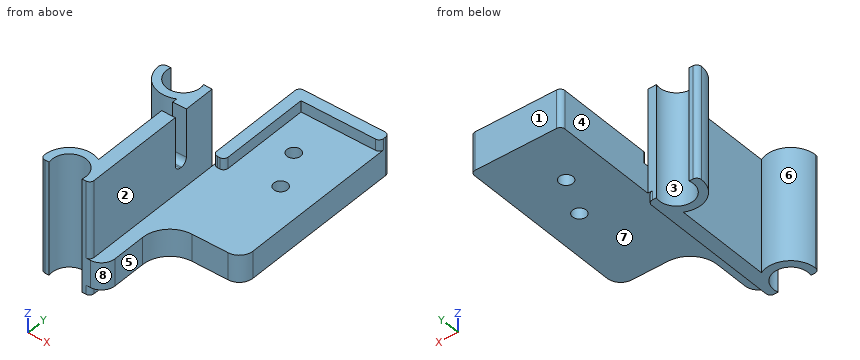
from build123d import *

# Parameters (mm, degrees)
SKETCH1_R           = 3.75
BOSS_EXTRUDE1_DEPTH = 25
FILLET1_R           = 2
SKETCH3_W           = 20
SKETCH3_H           = 19
CUT_EXTRUDE2_DEPTH  = 6
FILLET2_R           = 3
SKETCH7_W           = 32.058329052
SKETCH7_H           = 42.536839165
CUT_EXTRUDE5_DEPTH  = 25
SKETCH10_W          = 12.254265393
SKETCH10_H          = 5.748315633
SKETCH10_W_2        = 13.681746689
SKETCH10_H_2        = 5.503604554
CUT_EXTRUDE6_DEPTH  = 25
SKETCH11_W          = 6
SKETCH11_H          = 56.5
BOSS_EXTRUDE2_DEPTH = 20
CUT_EXTRUDE9_DEPTH  = 3
CUT_EXTRUDE11_DEPTH = 10
BOSS_EXTRUDE3_DEPTH = 2.5
FILLET5_R           = 3
FILLET6_R           = 1
SKETCH17_R          = 1.5
CUT_EXTRUDE12_DEPTH = 10


with BuildPart() as part:
    # Sketch1 → Boss-Extrude1 (new body)
    with BuildSketch(Plane.XY):
        with BuildLine():
            Line((-21, 16.5), (-21, -16.5))
            Line((-21, -16.5), (-16.5, -21))
            Line((-16.5, -21), (16.5, -21))
            Line((16.5, -21), (21, -16.5))
            Line((21, -16.5), (21, 16.5))
            Line((21, 16.5), (16.5, 21))
            Line((16.5, 21), (11.125, 21))
            Line((11.125, 21), (11.125, 18))
            Line((11.125, 18), (10.601020514, 18))
            ThreePointArc((10.601020514, 18), (11.610912703, 11.610912703), (18, 10.601020514))
            Line((18, 10.601020514), (18, -10.601020514))
            ThreePointArc((18, -10.601020514), (11.610912703, -11.610912703), (10.601020514, -18))
            Line((10.601020514, -18), (-10.601020514, -18))
            ThreePointArc((-10.601020514, -18), (-11.610912703, -11.610912703), (-18, -10.601020514))
            Line((-18, -10.601020514), (-18, 10.601020514))
            ThreePointArc((-18, 10.601020514), (-11.610912703, 11.610912703), (-10.601020514, 18))
            Line((-10.601020514, 18), (-11.125, 18))
            Line((-11.125, 18), (-11.125, 21))
            Line((-11.125, 21), (-16.5, 21))
            Line((-16.5, 21), (-21, 16.5))
        make_face()
        with Locations((-15.5, 15.5)):
            Circle(SKETCH1_R, mode=Mode.SUBTRACT)
        with Locations((15.5, 15.5)):
            Circle(SKETCH1_R, mode=Mode.SUBTRACT)
        with Locations((15.5, -15.5)):
            Circle(SKETCH1_R, mode=Mode.SUBTRACT)
        with Locations((-15.5, -15.5)):
            Circle(SKETCH1_R, mode=Mode.SUBTRACT)
    extrude(amount=BOSS_EXTRUDE1_DEPTH)

    # Fillet1
    fillet1_edges = [part.edges().sort_by_distance(p)[0] for p in [
        (-21, -16.5, 12.5),
        (-21, 16.5, 12.5),
        (-16.5, 21, 12.5),
        (-16.5, -21, 12.5),
    ]]
    fillet(fillet1_edges, radius=FILLET1_R)

    # Sketch3 → Cut-Extrude2 (cut)
    with BuildSketch(Plane(origin=(0, -21, 0), x_dir=(-1, 0, 0), z_dir=(0, -1, 0))):
        with Locations((0, -12.5)):
            Rectangle(SKETCH3_W, SKETCH3_H)
    extrude(amount=-CUT_EXTRUDE2_DEPTH, mode=Mode.SUBTRACT)

    # Fillet2
    fillet2_edges = [part.edges().sort_by_distance(p)[0] for p in [
        (10, -19.5, 22),
        (-10, -19.5, 3),
        (-10, -19.5, 22),
        (10, -19.5, 3),
    ]]
    fillet(fillet2_edges, radius=FILLET2_R)

    # Sketch7 → Cut-Extrude5 (cut)
    with BuildSketch(Plane.XY.offset(25)):
        with Locations((-6.029164526, 0.268419582)):
            Rectangle(SKETCH7_W, SKETCH7_H)
    extrude(amount=-CUT_EXTRUDE5_DEPTH, mode=Mode.SUBTRACT)

    # Sketch10 → Cut-Extrude6 (cut)
    with BuildSketch(Plane.XY.offset(25)):
        with Locations((14.872867304, 19.374157817)):
            Rectangle(SKETCH10_W, SKETCH10_H)
        with Locations((14.159126655, -19.251802277)):
            Rectangle(SKETCH10_W_2, SKETCH10_H_2)
    extrude(amount=-CUT_EXTRUDE6_DEPTH, mode=Mode.SUBTRACT)

    # Sketch11 → Boss-Extrude2 (add)
    with BuildSketch(Plane(origin=(21, 0, 0), x_dir=(0, 0, -1), z_dir=(1, 0, 0))):
        with Locations((-5, 11.75)):
            Rectangle(SKETCH11_W, SKETCH11_H)
    extrude(amount=BOSS_EXTRUDE2_DEPTH)

    # Sketch13 → Cut-Extrude9 (cut)
    with BuildSketch(Plane(origin=(21, 0, 0), x_dir=(0, 0, -1), z_dir=(1, 0, 0))):
        with BuildLine():
            Line((-25, 9.5), (-14.35, 9.5))
            ThreePointArc((-14.35, 9.5), (-13.395405845, 9.104594155), (-13, 8.15))
            Line((-13, 8.15), (-13, 7.85))
            ThreePointArc((-13, 7.85), (-13.395405845, 6.895405845), (-14.35, 6.5))
            Line((-14.35, 6.5), (-25, 6.5))
            Line((-25, 6.5), (-25, 9.5))
        make_face()
    extrude(amount=-CUT_EXTRUDE9_DEPTH, mode=Mode.SUBTRACT)

    # Sketch15 → Cut-Extrude11 (cut)
    with BuildSketch(Plane.XY.offset(8)):
        with BuildLine():
            Line((24, -16.5), (24, -6))
            ThreePointArc((24, -6), (25.757359313, -1.757359313), (30, 0))
            Line((30, 0), (41, 0))
            Line((41, 0), (41, -16.5))
            Line((41, -16.5), (24, -16.5))
        make_face()
    extrude(amount=-CUT_EXTRUDE11_DEPTH, mode=Mode.SUBTRACT)

    # Sketch16 → Boss-Extrude3 (add)
    with BuildSketch(Plane.XY.offset(8)):
        Polygon((21, 40), (41, 40), (41, 37.461788715), (23.538211285, 37.478793923), (23.538211285, 16.726527219), (21, 16.726527219), (21, 37.478793923), align=None)
    extrude(amount=BOSS_EXTRUDE3_DEPTH)

    # Fillet5
    fillet5_edges = [part.edges().sort_by_distance(p)[0] for p in [
        (41, 0, 5),
        (24, -16.5, 5),
    ]]
    fillet(fillet5_edges, radius=FILLET5_R)

    # Fillet6
    fillet6_edges = [part.edges().sort_by_distance(p)[0] for p in [
        (10.091673087, 16.5, 12.5),
        (10.091673087, -16.5, 12.5),
        (21, 16.5, 1),
        (21, -16.5, 1),
        (21, 40, 6.25),
        (41, 40, 6.25),
        (21, 16.726527219, 9.25),
        (23.538211285, 16.726527219, 9.25),
        (41, 37.461788715, 9.25),
        (21, -16.5, 16.5),
    ]]
    fillet(fillet6_edges, radius=FILLET6_R)

    # Sketch17 → Cut-Extrude12 (cut)
    with BuildSketch(Plane.XY.offset(8)):
        with Locations((29.574223118, 28.11574528)):
            Circle(SKETCH17_R)
        with Locations((33.574223119, 19.642947284)):
            Circle(SKETCH17_R)
    extrude(amount=-CUT_EXTRUDE12_DEPTH, mode=Mode.SUBTRACT)


solid = part.part
For this review, take the finished solid that the model builds, in its own axes (mm). Face numbers are marked on the shaded views. A direction names the side the tool comes from. Round coordinates to 2 decimals unless told otherwise and drop trailing zeros. Write each loop counter-clockwise with the first axis right and the second up, starting at its lowest first coordinate (ties: lowest second). Pieces come first, ordered by that corner, then holes. Notation, with made-up numbers: (34.25, -16.75) - (79.25, -16.75) arc R19 ccw to (79.25, -2.75) - close; hole circle Ø6 at (67.25, 51.25). An arc over 180 degrees is marked (long way). Use a Markdown table: item, result.
Q1. Clearance check with flat-ended pins moving along their axes: pin 1 (5 mm diameter, centred on x = 26, y = 7, fed in from -Z); pin 2 (2 mm diameter, centred on x = 17.5, z = 6, fed in from -Y); pin 3 (4.5 mm diameter, centred on x = 15.5, y = -15.5, fed in from +Z); pin 4 (3 mm diameter, centred on y = 20, z = 3.5, fed in from -X). State where each tip first meets the part, or that it passes through.
Derived:
| item | result |
|---|---|
| pin 1 | stops at z = 2 |
| pin 2 | stops at y = -13.25 |
| pin 3 | passes through |
| pin 4 | stops at x = 21 |
Q2. The part is to be moulded in two halves that separate along Y. For the marked faces 6, 7 and 8, say which applies: pulls with the +Y half, pulls with the -Y half, needs draft (parallel to the pull), parting line crosses it, or undercut.
Derived:
| item | result |
|---|---|
| face 6 | undercut |
| face 7 | needs draft |
| face 8 | pulls with the -Y half |
Q3. Machinability: for the marked faces 1, 2, 3, 4 and 5, which of the approach directions +Z, -Z, +X, -X, +Y, -Y give a long, thin tool a straight path to every point of the face, cutting with its end or side? Answer none if there is none.
Derived:
| item | result |
|---|---|
| face 1 | +Z, -Z, +X, -X, +Y |
| face 2 | +Z, +X, -Y |
| face 3 | +Z, -Z |
| face 4 | +Z, -Z, -X, +Y |
| face 5 | +Z, -Z, +X, -Y |
Q4. We need section C-C (z = 3.5). Give the boundary of the cut face in (x, y).
Derived:
| item | result |
|---|---|
| outline | (10, -15.5) arc R1 ccw to (11, -16.5) - (11.89, -16.5) arc R3.75 cw (long way) to (19.11, -16.5) - (21, -16.5) arc R3 ccw to (24, -13.5) - (24, -6) arc R6 cw to (30, 0) - (38, 0) arc R3 ccw to (41, 3) - (41, 39) arc R1 ccw to (40, 40) - (22, 40) arc R1 ccw to (21, 39) - (21, 16.5) - (19.11, 16.5) arc R3.75 cw (long way) to (11.89, 16.5) - (11, 16.5) arc R1 ccw to (10, 15.5) arc R5.5 ccw to (18, 10.6) - (18, -10.6) arc R5.5 ccw to start; hole circle Ø3 at (29.57, 28.12); hole circle Ø3 at (33.57, 19.64) |
Q5. Wall thickness on line 1 along Z through (x, y) = (38.5, 31.5); line 2 along Z through (x, y) = (22, 19.5); line 3 along Y through (x, z) = (35.5, 3): over which ranges is each line inside the solid? List them lowest first.
Derived:
| item | result |
|---|---|
| line 1 | z = 2 to 8 |
| line 2 | z = 2 to 10.5 |
| line 3 | y = 0 to 40 |
Q6. We need section A-A (x = 15.5). Give the boundary of the cut face in (y, z).
Derived:
| item | result |
|---|---|
| outline | (-11.75, 0) - (-10, 0) - (-10, 25) - (-11.75, 25) - close; (10, 0) - (11.75, 0) - (11.75, 25) - (10, 25) - close |
Q7. We need section D-D (x = 34). Give the boundary of the cut face in (y, z).
Derived:
| item | result |
|---|---|
| outline | (0, 2) - (18.2, 2) - (18.2, 8) - (0, 8) - close; (21.08, 2) - (40, 2) - (40, 10.5) - (37.47, 10.5) - (37.47, 8) - (21.08, 8) - close |
Q8. We need section B-B (z = 17). Give the boundary of the cut face in (x, y), plus the area to 3 significant figures.
Derived:
| item | result |
|---|---|
| outline | (10, -15.5) arc R1 ccw to (11, -16.5) - (11.89, -16.5) arc R3.75 cw (long way) to (19.11, -16.5) - (20, -16.5) arc R1 ccw to (21, -15.5) - (21, 6.5) - (18, 6.5) - (18, -10.6) arc R5.5 ccw to start; (10, 15.5) arc R5.5 ccw to (18, 10.6) - (18, 9.5) - (21, 9.5) - (21, 16.5) - (19.11, 16.5) arc R3.75 cw (long way) to (11.89, 16.5) - (11, 16.5) arc R1 ccw to start |
| area | 120 mm2 |
